Could you check a few things on this model? Use its own coordinates, in mm. A direction names the side the tool comes from. Give positions to 0.01 mm unless a question says otherwise; leave off trailing zeros. Order: outer loops, then holes, each group sorted by start corner. A loop starts at its lowest first (then second) coordinate and runs counter-clockwise, first axis right, second up. Notation, with made-up numbers: (86, 23) - (130, 23) arc R24 ccw to (130, 50) - close; hole circle Ø11 at (45, -36). An arc over 180 degrees is marked (long way). One line per question, with ' | ' between items. Start each with the question number.
1. I need wall thicknesses on probe 1 along Y at (x, z) = (0, 0.95); probe 2 along Z at (x, y) = (-4.5, 14.5); probe 3 along Y at (x, z) = (-1, -3.5). Which ranges of each line are inside material? Lowest first, please. Write a range as from..to.
2. Imagine slicing it at A-A (x = 0). Give the number of separate pieces and of enclosed holes in the cut face, and give its area (4 significant figures).
3. Which directions (+Z, -Z, +X, -X, +Y, -Y) give clear straight access to the entire face, cutting with the end or side of a thin tool? Please do faces 1 (the flat face through (5, 0, -15)), 2 (the flat face through (-0.3, -8.3, 0)).
4. Imagine slicing it at C-C (z = 2.75). Please give me the cut outline in (x, y), and give its area (3 significant figures).
5. If we mould it in two halves opening along X, with no side actions, what happens to faces 3 (the flat face through (-0.3, -8.3, 2)), 4 (the cylindrical face through (-1.73, -7.81, 3.23)), 5 (the cylindrical face through (0, -12, 1))? For each: released by +X, released by -X, zero draft, split by the parting line, or undercut.
6. For P1, Ø5, axis at x = 13, y = -9, coming from the -Z side; P2, Ø12, axis at x = -7, z = -7, coming from the -Y side; P3, Ø6.5, axis at x = 0, y = -14, coming from the +Z side, each with a flat end and sliding along its axis, tell me the tip position at first contact or that it passes through.
```python
from build123d import *

# Parameters (mm, degrees)
SKETCH_1_R         = 19.75
EXTRUDE_1_DEPTH    = 2
SKETCH_2_R         = 8
EXTRUDE_2_DEPTH    = 3
EXTRUDE_START      = 15
SKETCH_3_R         = 8
EXTRUDE_3_DEPTH    = 15
HOLE_WIZARD_M8_1_D = 8
HOLE_WIZARD_M4_1_D = 4
CHAMFER_1_SIZE     = 0.5


with BuildPart() as part:
    # 草图1 → 凸台-拉伸1 (new body)
    with BuildSketch(Plane.XY):
        Circle(SKETCH_1_R)
    extrude(amount=EXTRUDE_1_DEPTH)

    # 草图2 → 凸台-拉伸2 (add)
    with BuildSketch(Plane.XY.offset(2)):
        Circle(SKETCH_2_R)
    extrude(amount=EXTRUDE_2_DEPTH)

    # 草图3 → 凸台-拉伸3 (add)
    with BuildSketch(Plane(origin=(0, 0, 0), x_dir=(-1, 0, 0), z_dir=(0, 0, -1)).offset(EXTRUDE_START)):
        with Locations(Location((0, 0, 0), (0, 0, 180))):
            Circle(SKETCH_3_R)
    extrude(amount=-EXTRUDE_3_DEPTH)

    # M8 螺纹孔1 (through all)
    with Locations(Plane.XY.offset(5)):
        with Locations((0, 0)):
            Hole(HOLE_WIZARD_M8_1_D / 2)

    # M4 螺纹孔1 (through all)
    with Locations(Plane.XY.offset(2)):
        with Locations((0, 14), (0, -14), (-14, 0), (14, 0)):
            Hole(HOLE_WIZARD_M4_1_D / 2)

    # 倒角1
    chamfer_1_edges = [part.edges().sort_by_distance(p)[0] for p in [
        (-8, 0, -15),
        (4, 0, 5),
        (4, 0, -15),
        (-19.75, 0, 0),
        (-19.75, 0, 2),
        (-8, 0, 5),
    ]]
    chamfer(chamfer_1_edges, length=CHAMFER_1_SIZE)


solid = part.part
```
Results found:
1) probe 1: y = -19.75..-16, -12..-4, 4..12, 16..19.75 | probe 2: z = 0..2 | probe 3: y = -7.94..-3.87, 3.87..7.94
2) separate pieces: 4 | enclosed holes: 0 | area: 189.5 mm2
3) face 1: -Z, +X, -X, +Y, -Y | face 2: -Z
4) outline: circle Ø16 at (0, 0); hole circle Ø8 at (0, 0) | area: 151 mm2
5) face 3: zero draft | face 4: split by the parting line | face 5: undercut
6) P1: stops at z = 0 | P2: stops at y = -7.94 | P3: stops at z = 2
